The listing builds one solid part. Answer for the finished solid, in the listing's coordinates (mm). A direction names the side the tool comes from. Round coordinates to 2 decimals unless told otherwise and drop trailing zeros. Loops run counter-clockwise (first coordinate to the right, second up) from the corner with the lowest first, then second, coordinate; pieces in that order, holes last. Notation, with made-up numbers: (-12.75, 75.25) - (7.25, 75.25) arc R5 ccw to (7.25, 80.25) - close; hole circle Ø9 at (-18, 32). An arc over 180 degrees is marked (long way). Write item = value, one per line. Start each with the question number.
1) Straight lines are drawn through the part: line 1 along X through (y, z) = (32, -4.25); line 2 along Y through (x, z) = (-24.5, 0); line 3 along Y through (x, z) = (22.25, 0). For each, find the intervals that lie inside material, in ascending order.
2) Section D-D, the plane x = 28 is taken. Determine the outline of the cut face in (y, z) (3 decimals), and give its area (3 significant figures).
3) For a pull along X with two mould halves and no side action, classify faces 6 (the flat face through (12.7, -1, 0)), 7 (the flat face through (0, 52, -10.439)), 8 (the conical face through (-24.5, 46.6, 1)), 9 (the flat face through (0, 50, -12.7)) as released by +X, released by -X, zero draft, split by the parting line, or undercut.
4) Section C-C, the plane x = -24 is taken. Determine the outline of the cut face in (y, z) (1 decimal).
5) Section A-A, the plane x = 7.5 is taken. Determine the outline of the cut face in (y, z) (3 decimals).
6) Given pin 1 Ø2 at (x, z) = (4.5, 6) entering from +Y; pin 2 Ø8 at (y, z) = (30.5, 4) entering from -X; pin 3 Ø1.5 at (x, z) = (-23.5, -1) entering from -Y, each flat-ended and moving along its own axis, determine where each tip first touches the part or whether it passes through.
7) Section B-B, the plane y = 29.5 is taken. Determine the outline of the cut face in (x, z) (3 decimals), and give its area (3 significant figures).
8) A tool of negligible diameter and unlimited length cuts with its end or side. For faces 1 (the flat face through (7, 52, -10.185)), 2 (the flat face through (-11.201, 33, 0)), 3 (the flat face through (-19.05, 54, 0)), 4 (the flat face through (19.05, 10, 0)), 5 (the flat face through (-12.7, -1, 0)), from which of +Z, -Z, +X, -X, +Y, -Y can it reach the whole face along a straight path? Write none if from no direction.
from build123d import *

# Parameters (mm, degrees)
SKETCH1_W               = 25.4
SKETCH1_H               = 25.4
BOSS_EXTRUDE1_DEPTH     = 67.056
SKETCH4_W               = 25.4
SKETCH4_H               = 25.4
BOSS_EXTRUDE4_DEPTH     = 3.175
SKETCH5_R               = 30.1625
CUT_EXTRUDE1_DEPTH      = 3.175
SKETCH7_R               = 9.525
BOSS_EXTRUDE6_DEPTH     = 19.05
BOSS_EXTRUDE6_TAPER     = 10
SKETCH8_R               = 1.905
CUT_EXTRUDE2_DEPTH      = 12.7
LPATTERN1_COUNT         = 2
LPATTERN1_PITCH         = 44.45
MIRROR2_COPY_1_SKETCH_R = 9.525
MIRROR2_COPY_1_DEPTH    = 19.05
MIRROR2_COPY_1_TAPER    = 10
MIRROR2_COPY_2_SKETCH_R = 1.905
MIRROR2_COPY_2_DEPTH    = 12.7
CHAMFER1_SIZE           = 6.35


with BuildPart() as part:
    # Sketch1 → Boss-Extrude1 (new body)
    with BuildSketch(Plane(origin=(0, 0, 0), x_dir=(1, 0, 0), z_dir=(0, 1, 0))):
        Rectangle(SKETCH1_W, SKETCH1_H)
        with BuildLine():
            Line((4.7625, -10.1854), (8.329805012, -10.1854))
            Line((8.329805012, -10.1854), (8.376905012, -10.154))
            Line((8.376905012, -10.154), (9.416515139, -10.154))
            ThreePointArc((9.416515139, -10.154), (9.501675056, -10.1507417), (9.586332782, -10.140948982))
            Line((9.586332782, -10.140948982), (9.615351798, -10.140948982))
            ThreePointArc((9.615351798, -10.140948982), (10.251622353, -9.784337345), (10.504, -9.1))
            Line((10.504, -9.1), (10.504, -8.735936675))
            Line((10.504, -8.735936675), (11.2014, -8.271003341))
            Line((11.2014, -8.271003341), (11.2014, 8.271003341))
            Line((11.2014, 8.271003341), (8.329805012, 10.1854))
            Line((8.329805012, 10.1854), (4.7625, 10.1854))
            Line((4.7625, 10.1854), (4.7625, 10.4394))
            Line((4.7625, 10.4394), (-4.7625, 10.4394))
            Line((-4.7625, 10.4394), (-4.7625, 10.1854))
            Line((-4.7625, 10.1854), (-8.329805012, 10.1854))
            Line((-8.329805012, 10.1854), (-11.2014, 8.271003341))
            Line((-11.2014, 8.271003341), (-11.2014, -8.271003341))
            Line((-11.2014, -8.271003341), (-10.504, -8.735936675))
            Line((-10.504, -8.735936675), (-10.504, -9.1))
            ThreePointArc((-10.504, -9.1), (-10.251622353, -9.784337345), (-9.615351798, -10.140948982))
            Line((-9.615351798, -10.140948982), (-9.586332782, -10.140948982))
            ThreePointArc((-9.586332782, -10.140948982), (-9.501675056, -10.1507417), (-9.416515139, -10.154))
            Line((-9.416515139, -10.154), (-8.376905012, -10.154))
            Line((-8.376905012, -10.154), (-8.329805012, -10.1854))
            Line((-8.329805012, -10.1854), (-4.7625, -10.1854))
            Line((-4.7625, -10.1854), (-4.7625, -10.4394))
            Line((-4.7625, -10.4394), (4.7625, -10.4394))
            Line((4.7625, -10.4394), (4.7625, -10.1854))
        make_face(mode=Mode.SUBTRACT)
    extrude(amount=BOSS_EXTRUDE1_DEPTH)

    # Sketch4 → Boss-Extrude4 (add)
    with BuildSketch(Plane(origin=(0, 0, 0), x_dir=(-1, 0, 0), z_dir=(0, -1, 0))):
        Rectangle(SKETCH4_W, SKETCH4_H)
    extrude(amount=BOSS_EXTRUDE4_DEPTH)

    # Sketch5 → Cut-Extrude1 (cut)
    with BuildSketch(Plane(origin=(0, 0, -12.7), x_dir=(-1, 0, 0), z_dir=(0, 0, -1))):
        with Locations((0, 11.43)):
            Circle(SKETCH5_R)
    cut_extrude1 = extrude(amount=-CUT_EXTRUDE1_DEPTH, mode=Mode.SUBTRACT)

    # Mirror1: Cut-Extrude1 across plane
    add(cut_extrude1.mirror(Plane.XY), mode=Mode.SUBTRACT)

    # Sketch7 → Boss-Extrude6 (add)
    with BuildSketch(Plane(origin=(12.7, 0, 0), x_dir=(0, 0, -1), z_dir=(1, 0, 0))):
        with Locations((0, 9.525)):
            Circle(SKETCH7_R)
    boss_extrude6 = extrude(amount=BOSS_EXTRUDE6_DEPTH, taper=BOSS_EXTRUDE6_TAPER)

    # Sketch8 → Cut-Extrude2 (cut)
    with BuildSketch(Plane(origin=(31.75, 0, 0), x_dir=(0, 0, -1), z_dir=(1, 0, 0))):
        with Locations((0, 9.525)):
            Circle(SKETCH8_R)
    cut_extrude2 = extrude(amount=-CUT_EXTRUDE2_DEPTH, mode=Mode.SUBTRACT)

    # LPattern1: Boss-Extrude6, Cut-Extrude2 ×2
    with Locations(*[(0, i * LPATTERN1_PITCH, 0) for i in range(1, LPATTERN1_COUNT)]):
        add(boss_extrude6)
        add(cut_extrude2, mode=Mode.SUBTRACT)

    # Mirror2: Boss-Extrude6, Cut-Extrude2 across plane
    add(boss_extrude6.mirror(Plane(origin=(0, 0, 0), x_dir=(0, 0, 1), z_dir=(1, 0, 0))))
    add(cut_extrude2.mirror(Plane(origin=(0, 0, 0), x_dir=(0, 0, 1), z_dir=(1, 0, 0))), mode=Mode.SUBTRACT)

    # Mirror2 copy 1 sketch → Mirror2 copy 1 (add)
    with BuildSketch(Plane(origin=(-12.7, 44.45, 0), x_dir=(0, 0, -1), z_dir=(-1, 0, 0))):
        with Locations((0, -9.525)):
            Circle(MIRROR2_COPY_1_SKETCH_R)
    extrude(amount=MIRROR2_COPY_1_DEPTH, taper=MIRROR2_COPY_1_TAPER)

    # Mirror2 copy 2 sketch → Mirror2 copy 2 (cut)
    with BuildSketch(Plane(origin=(-31.75, 44.45, 0), x_dir=(0, 0, -1), z_dir=(-1, 0, 0))):
        with Locations((0, -9.525)):
            Circle(MIRROR2_COPY_2_SKETCH_R)
    extrude(amount=-MIRROR2_COPY_2_DEPTH, mode=Mode.SUBTRACT)

    # Chamfer1
    # the kernel refuses this chamfer: 6.35 mm, written as the material it takes off along each edge
    with BuildSketch(Plane(origin=(-29.030186974, 67.056, 12.7), x_dir=(0, -0.9996219169112968, 0.027495876610586455), z_dir=(1, 0, 0))) as chamfer1_piece_1:
        Polygon((CHAMFER1_SIZE * 0.999621916911, CHAMFER1_SIZE * 0.0274958766106), (-CHAMFER1_SIZE * 0.0274958766106, CHAMFER1_SIZE * 0.999621916911), (0, 0), align=None)
    extrude(amount=58.060373947, mode=Mode.SUBTRACT)
    with BuildSketch(Plane(origin=(29.030186974, 67.056, -12.7), x_dir=(0, 0.027495876610585654, 0.9996219169112966), z_dir=(-1, 0, 0))) as chamfer1_piece_2:
        Polygon((CHAMFER1_SIZE * 0.999621916911, -CHAMFER1_SIZE * 0.0274958766106), (-CHAMFER1_SIZE * 0.0274958766106, -CHAMFER1_SIZE * 0.999621916911), (0, 0), align=None)
    extrude(amount=58.060373947, mode=Mode.SUBTRACT)


solid = part.part
Geometry check:
q1.line_1 = -12.7 to -11.2, 11.2 to 12.7
q1.line_2 = 2.08 to 7.62, 11.43 to 16.97, 46.53 to 52.07, 55.88 to 61.42
q1.line_3 = 1.68 to 7.62, 11.43 to 17.37, 46.13 to 52.07, 55.88 to 61.82
q2.outline = circle Ø13.654 at (9.525, 0); circle Ø13.654 at (53.975, 0); hole circle Ø3.81 at (9.525, 0); hole circle Ø3.81 at (53.975, 0)
q2.area = 270 mm2
q3.face_6 = released by +X
q3.face_7 = undercut
q3.face_8 = released by -X
q3.face_9 = zero draft
q4.outline = circle Ø15.1 at (9.5, 0); circle Ø15.1 at (54, 0); hole circle Ø3.8 at (9.5, 0); hole circle Ø3.8 at (54, 0)
q5.outline = (-3.175, -9.525) - (0, -9.525) - (0, 9.525) - (-3.175, 9.525) - close; (40.645, -12.7) - (60.706, -12.7) - (63.221, -10.185) - (40.645, -10.185) - close; (40.645, 10.185) - (63.221, 10.185) - (60.706, 12.7) - (40.645, 12.7) - close
q6.pin_1 = 0
q6.pin_2 = -12.7
q6.pin_3 = 1.81
q7.outline = (-12.7, -9.525) - (-9.32, -9.525) - (-11.201, -8.271) - (-11.201, 8.271) - (-10.504, 8.736) - (-10.504, 9.1) arc R1.054 cw to (-10.415, 9.525) - (-12.7, 9.525) - close; (9.32, -9.525) - (12.7, -9.525) - (12.7, 9.525) - (10.415, 9.525) arc R1.054 cw to (10.504, 9.1) - (10.504, 8.736) - (11.201, 8.271) - (11.201, -8.271) - close
q7.area = 60.9 mm2
q8.face_1 = +Y, -Y
q8.face_2 = +Y
q8.face_3 = -X
q8.face_4 = +X
q8.face_5 = -X, -Y
